The figure shows three views and two pictorial views of one solid part (mm, origin at its lowest corner). Answer the questions. A direction names the side the tool comes from. Round coordinates to 2 decimals unless told otherwise and drop trailing zeros. Write each loop counter-clockwise with the first axis right and the second up, starting at its lowest first coordinate (ties: lowest second). Pieces come first, ordered by that corner, then holes.
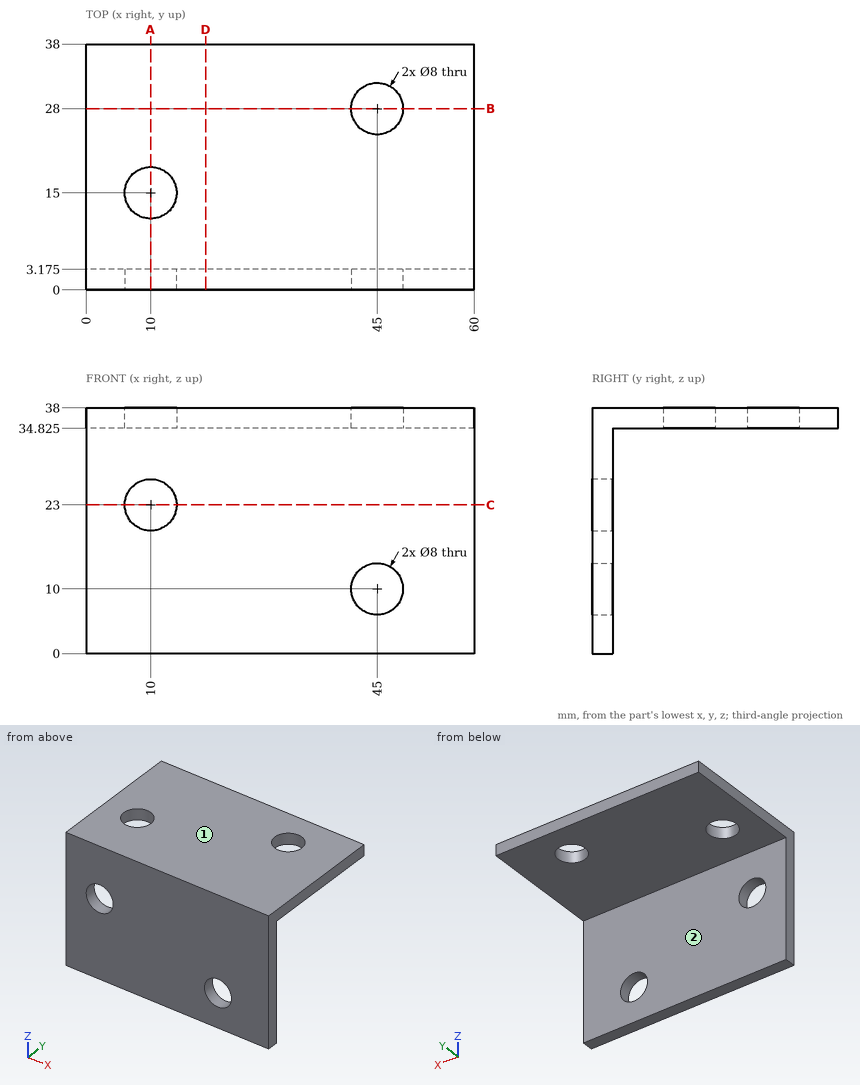
Q1. Straight lines are drawn through the part: probe 1 along Y at (x, z) = (10, 37.05); probe 2 along Y at (x, z) = (45.5, 18.5) (3 decimals); probe 3 along Z at (x, y) = (5, 9.5) (3 decimals). For each, find the intervals that lie inside material, in ascending order.
Verdict:
probe 1: y = 0 to 11, 19 to 38
probe 2: y = 0 to 3.175
probe 3: z = 34.825 to 38
Q2. Section D-D (x = 18.5) is taken. Determine the outline of the cut face in (y, z) (3 decimals).
Verdict:
outline: (0, 0) - (3.175, 0) - (3.175, 34.825) - (38, 34.825) - (38, 38) - (0, 38) - close
Q3. Flat-ended cylindrical pins translate along their axes: pin 1 Ø13 at (x, z) = (10, 23) entering from -Y; pin 2 Ø10.5 at (x, z) = (24.5, 17.5) entering from +Y (3 decimals); pin 3 Ø4 at (x, y) = (27.5, 33.5) entering from -Z (3 decimals). Find the tip coordinate at first contact, or state that the pin passes through.
Verdict:
pin 1: stops at y = 0
pin 2: stops at y = 3.175
pin 3: stops at z = 34.825
Q4. Section C-C (z = 23) is taken. Determine the outline of the cut face in (x, y) (3 decimals), then the cut area to 3 significant figures.
Verdict:
outline: (0, 0) - (6, 0) - (6, 3.175) - (0, 3.175) - close; (14, 0) - (60, 0) - (60, 3.175) - (14, 3.175) - close
area: 165 mm2
Q5. Section A-A (x = 10) is taken. Determine the outline of the cut face in (y, z) (3 decimals), then the cut area to 3 significant figures.
Verdict:
outline: (0, 0) - (3.175, 0) - (3.175, 19) - (0, 19) - close; (0, 27) - (3.175, 27) - (3.175, 34.825) - (11, 34.825) - (11, 38) - (0, 38) - close; (19, 34.825) - (38, 34.825) - (38, 38) - (19, 38) - close
area: 180 mm2
Q6. Section B-B (y = 28) is taken. Determine the outline of the cut face in (x, z) (3 decimals), then the cut area to 3 significant figures.
Verdict:
outline: (0, 34.825) - (41, 34.825) - (41, 38) - (0, 38) - close; (49, 34.825) - (60, 34.825) - (60, 38) - (49, 38) - close
area: 165 mm2
Q7. Which of the six approach directions +Z, -Z, +X, -X, +Y, -Y give full straight-line access (tool end or side, diameter ignored) to the marked faces 1 and 2?
Verdict:
face 1: +Z, +X, -X, +Y, -Y
face 2: -Z, +X, -X, +Y
